```python
from build123d import *

# Parameters (mm, degrees)
SKETCH1_R           = 4.7625
SKETCH1_R_2         = 2.3749
BOSS_EXTRUDE1_DEPTH = 4.7625
FILLET1_R           = 2.54


with BuildPart() as part:
    # Sketch1 → Boss-Extrude1 (new body, symmetric)
    with BuildSketch(Plane(origin=(0, 0, 0), x_dir=(1, 0, 0), z_dir=(0, 1, 0))):
        with BuildLine():
            ThreePointArc((-15.875, 0), (0, -15.875), (15.875, 0))
            ThreePointArc((15.875, 0), (8.330712377, 6.107698439), (4.7752, 15.139785004))
            ThreePointArc((4.7752, 15.139785004), (0, 15.875), (-4.7752, 15.139785004))
            ThreePointArc((-4.7752, 15.139785004), (-8.330712377, 6.107698439), (-15.875, 0))
        make_face()
        Circle(SKETCH1_R, mode=Mode.SUBTRACT)
        with Locations((0, 9.525)):
            Circle(SKETCH1_R_2, mode=Mode.SUBTRACT)
    extrude(amount=BOSS_EXTRUDE1_DEPTH, both=True)

    # Fillet1
    fillet1_edges = [part.edges().sort_by_distance(p)[0] for p in [
        (0, 4.7625, 15.875),
        (8.330712377, 4.7625, -6.107698439),
        (0, 4.7625, -15.875),
        (8.330712377, -4.7625, -6.107698439),
        (0, -4.7625, 15.875),
        (-8.330712377, -4.7625, -6.107698439),
        (0, -4.7625, -15.875),
        (-8.330712377, 4.7625, -6.107698439),
    ]]
    fillet(fillet1_edges, radius=FILLET1_R)


solid = part.part
```
Work out the finished part from the listing and answer in its coordinate system (mm). Give positions to 0.01 mm unless a question says otherwise; leave off trailing zeros. Write each loop counter-clockwise with the first axis right and the second up, starting at its lowest first coordinate (ties: lowest second). Pieces come first, ordered by that corner, then holes.
(1) Straight lines are drawn through the part: line 1 (Z direction, x = 0, y = -0.75) (1 decimal); line 2 (X direction, y = -4.5, z = 4); line 3 (Z direction, x = -4, y = -1.75). For each, find the intervals that lie inside material, in ascending order.
Final values:
line 1: z = -15.9 to -11.9, -7.2 to -4.8, 4.8 to 15.9
line 2: x = -13.9 to -2.58, 2.58 to 13.9
line 3: z = -15.36 to -2.58, 2.58 to 15.36
(2) The part is cut by section C-C on y = 1.25. Count the separate pieces of the cut face and the enclosed holes in it, plus the area to 3 significant figures.
Final values:
separate pieces: 1
enclosed holes: 2
area: 561 mm2
(3) The part is cut by section A-A on x = 0. Write down the section's boundary in (y, z) (1 decimal).
Final values:
outline: (-4.8, -13.3) arc R2.5 ccw to (-2.2, -15.9) - (2.2, -15.9) arc R2.5 ccw to (4.8, -13.3) - (4.8, -11.9) - (-4.8, -11.9) - close; (-4.8, -7.2) - (4.8, -7.2) - (4.8, -4.8) - (-4.8, -4.8) - close; (-4.8, 4.8) - (4.8, 4.8) - (4.8, 13.3) arc R2.5 ccw to (2.2, 15.9) - (-2.2, 15.9) arc R2.5 ccw to (-4.8, 13.3) - close
(4) The part is cut by section B-B on y = 4. Write down the section's boundary in (x, z) (1 decimal), plus the area to 3 significant figures.
Final values:
outline: (-15.1, 0.5) arc R19.8 cw to (-4.1, -14.6) arc R15.1 ccw to (4.1, -14.6) arc R19.8 cw to (15.1, 0.5) arc R15.1 ccw to start; hole circle Ø9.5 at (0, 0); hole circle Ø4.7 at (0, -9.5)
area: 492 mm2
(5) Flat-ended cylindrical pins translate along their axes: pin 1 Ø1.5 at (y, z) = (2, -10) entering from +X; pin 2 Ø3 at (x, y) = (9, 1.5) entering from -Z; pin 3 Ø2 at (y, z) = (-3, -8) entering from +X. Find the tip coordinate at first contact, or state that the pin passes through.
Final values:
pin 1: stops at x = 6.46
pin 2: stops at z = -7.34
pin 3: stops at x = 7.63
(6) The mould has two halves that part along Z. Classify faces 1 (the flat face through (0, 4.762, 6)), 2 (the cylindrical face through (-3.78, -0.07, 2.9)), 3 (the cylindrical face through (-0.35, 0.03, 15.87)): pulls with the +Z half, pulls with the -Z half, needs draft (parallel to the pull), parting line crosses it, or undercut.
Final values:
face 1: needs draft
face 2: undercut
face 3: pulls with the +Z half
